Job drawing, mm, ordinate dimensions from the low corner. One solid piece. A direction names the side the tool comes from. Round coordinates to 2 decimals unless told otherwise and drop trailing zeros. Write each loop counter-clockwise with the first axis right and the second up, starting at its lowest first coordinate (ties: lowest second). Pieces come first, ordered by that corner, then holes.
1) Which spindle directions (+Z, -Z, +X, -X, +Y, -Y) get a long thin tool onto all of the face, cutting with end or side? Do the marked faces 4 and 5. Say none if no direction does.
2) Pull direction X, two halves, no side cores. Call the marked faces 1, 2 and 3: +X half, -X half, draft (parallel to the pull), parting line (faces both ways), or undercut.
3) Flat gauge pins, fed straight in: pin 1 (3 mm diameter, centred on x = 35.56, z = 30.8, fed in from -Y); pin 2 (4 mm diameter, centred on x = 10, z = 40, fed in from +Y); pin 3 (13.5 mm diameter, centred on x = 19.5, z = 40.5, fed in from +Y); pin 4 (1.4 mm diameter, centred on x = 12.5, z = 60.5, fed in from -Y). Where does each tip first touch, or does it go through?
4) Drill centre lines: L1, parallel to Z at x = 10, y = 12.75; L2, parallel to X at y = 12.25, z = 53; L3, parallel to Y at x = 7, z = 38.5. Where is each one in solid material? Low to high.
5) Saw through at C-C on y = 6. Count the separate pieces of the cut face and the enclosed holes in it.
6) Saw through at A-A on y = 11.5. Write the cut outline in (x, z).
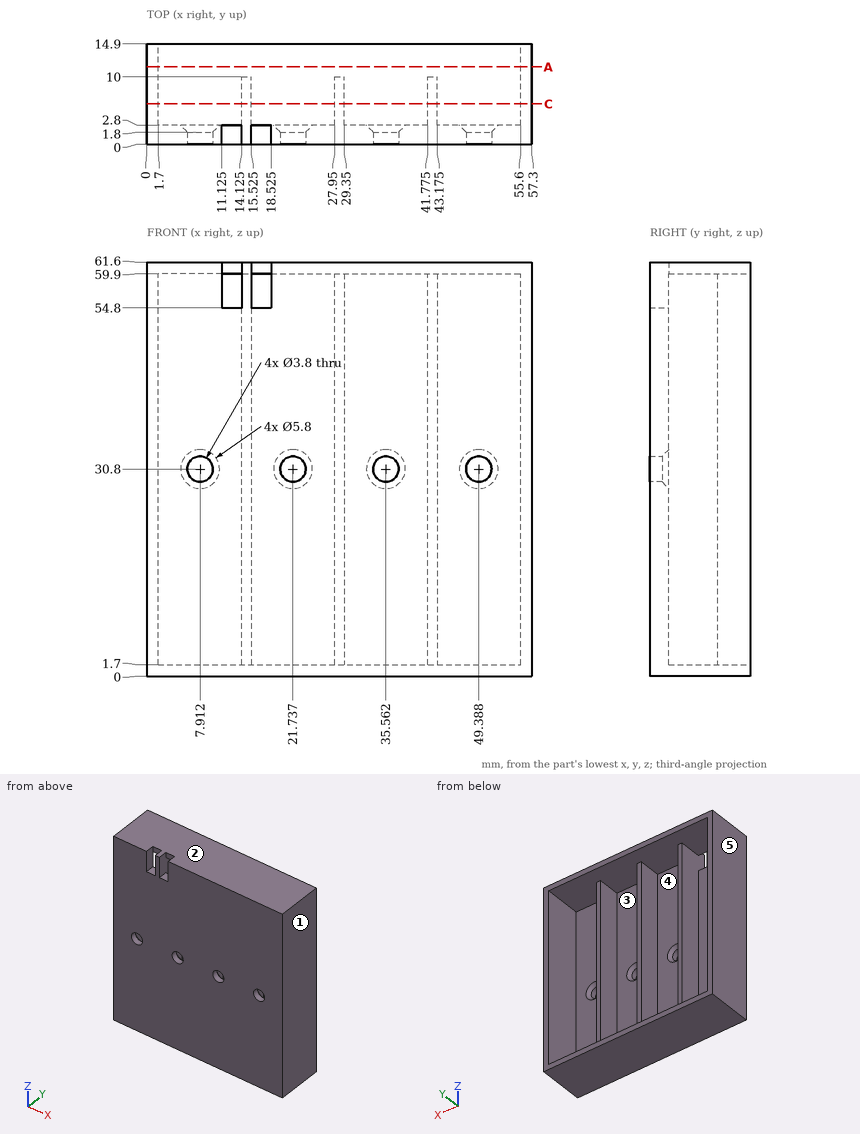
Completed:
1. face 4: +Y
1. face 5: +Z, -Z, -X, +Y, -Y
2. face 1: +X half
2. face 2: draft
2. face 3: undercut
3. pin 1: passes through
3. pin 2: stops at y = 2.8
3. pin 3: stops at y = 10
3. pin 4: stops at y = 2.8
4. L1: z = 0 to 1.7, 59.9 to 61.6
4. L2: x = 0 to 1.7, 55.6 to 57.3
4. L3: y = 0 to 2.8
5. separate pieces: 1
5. enclosed holes: 4
6. outline: (0, 0) - (57.3, 0) - (57.3, 61.6) - (0, 61.6) - close; hole (1.7, 1.7) - (55.6, 1.7) - (55.6, 59.9) - (1.7, 59.9) - close
